Build history of the part. All positions in model axes, mm. Coordinates: 2 decimals unless noted, no trailing zeros. Loops run counter-clockwise (first coordinate to the right, second up) from the corner with the lowest first, then second, coordinate; pieces in that order, holes last. Notation, with made-up numbers: (40, 89.5) - (56, 89.5) arc R22 ccw to (56, 118.5) - close; hole circle Ø7 at (-28.75, -19.5). An arc over 180 degrees is marked (long way). One line per item, written item: value.
```python
from build123d import *

# Parameters (mm, degrees)
F3_DEPTH = 25


with BuildPart() as f1:
    # F0 (on Top) → F1 (revolve)
    with BuildSketch(Plane.XY):
        with BuildLine():
            Line((1.5, 5.3077938069), (1.5, 0))
            Line((1.5, 0), (9.45, 0))
            Line((9.45, 0), (9.676587279, 2.58990445))
            ThreePointArc((9.676587279, 2.58990445), (9.0292938758, 4.4967693259), (7.1861005338, 5.3077938069))
            Line((7.1861005338, 5.3077938069), (1.5, 5.3077938069))
        make_face()
    revolve(axis=Axis((0, 4.3452630795, 0), (0, 1, 0)))

    # F2 (on face) → F3 (cut)
    with BuildSketch(Plane.XZ):
        with BuildLine():
            ThreePointArc((9.45, 0), (9.4496021647, -0.0867117579), (9.4484086923, -0.1734162148))
            Line((9.4484086923, -0.1734162148), (11.2557578832, -0.2065883251))
            Line((11.2557578832, -0.2065883251), (11.2557578832, 0))
            Line((11.2557578832, 0), (11.2557578832, 0.2065883251))
            Line((11.2557578832, 0.2065883251), (9.4484086923, 0.1734162148))
            ThreePointArc((9.4484086923, 0.1734162148), (9.4496021647, 0.0867117579), (9.45, 0))
        make_face()
        with BuildLine():
            ThreePointArc((1.5, 0), (1.4999368515, -0.0137637711), (1.4997474115, -0.0275263833))
            Line((1.4997474115, -0.0275263833), (9.4484086923, -0.1734162148))
            ThreePointArc((9.4484086923, -0.1734162148), (9.4496021647, -0.0867117579), (9.45, 0))
            ThreePointArc((9.45, 0), (9.4496021647, 0.0867117579), (9.4484086923, 0.1734162148))
            Line((9.4484086923, 0.1734162148), (1.4997474115, 0.0275263833))
            ThreePointArc((1.4997474115, 0.0275263833), (1.4999368515, 0.0137637711), (1.5, 0))
        make_face()
    extrude(amount=-F3_DEPTH, mode=Mode.SUBTRACT)


solid = f1.part
```
Item 1: Pull direction Z, two halves, no side cores. Call faces 1 (the face through (-1.5, 2.62, -0.07)), 2 (the face through (-9.48, 0.45, -0.41)), 3 (the face through (-2, 0, 0)): released by +Z, released by -Z, zero draft, split by the parting line, or undercut.
Check result:
face 1: undercut
face 2: split by the parting line
face 3: zero draft
Item 2: Drop flat-ended pins along their axis: P1, Ø3, axis at x = -1.5, y = 2, coming from the -Z side; P2, Ø1, axis at x = 3.5, y = 0.5, coming from the -Z side. Give the stop position or say it passes through.
Check result:
P1: stops at z = -9.68
P2: stops at z = -9.01
Item 3: Cut at D-D, the plane y = 4.1. Write the cut outline in (x, z), then the cut area to 3 significant figures.
Check result:
outline: (1.5, -0.03) arc R1.5 cw (long way) to (1.5, 0.03) - (9.32, 0.17) arc R9.33 ccw (long way) to (9.32, -0.17) - close
area: 265 mm^2
Item 4: Probe probe 1 along Z at (x, y) = (0, 3); probe 2 along Z at (x, y) = (0, 3.55); probe 3 along X at (y, z) = (1.75, -1). List the from-to ranges inside material, lowest first. Write a range as from..to.
Check result:
probe 1: z = -9.68..-1.5, 1.5..9.68
probe 2: z = -9.57..-1.5, 1.5..9.57
probe 3: x = -9.55..-1.12, 1.12..9.55
Item 5: Cut at A-A, the plane x = 0. Write the cut outline in (y, z).
Check result:
outline: (0, -9.45) - (2.59, -9.68) arc R2.5 ccw to (5.31, -7.19) - (5.31, -1.5) - (0, -1.5) - close; (0, 1.5) - (5.31, 1.5) - (5.31, 7.19) arc R2.5 ccw to (2.59, 9.68) - (0, 9.45) - close
Item 6: Cut at B-B, the plane y = 3.05. Write the cut outline in (x, z).
Check result:
outline: (1.5, -0.03) arc R1.5 cw (long way) to (1.5, 0.03) - (9.67, 0.18) arc R9.67 ccw (long way) to (9.67, -0.18) - close
Item 7: Cut at C-C, the plane y = 0.3. Write the cut outline in (x, z).
Check result:
outline: (1.5, -0.03) arc R1.5 cw (long way) to (1.5, 0.03) - (9.47, 0.17) arc R9.48 ccw (long way) to (9.47, -0.17) - close
